Geometry: final body of the model. Coordinates: model frame, mm. A direction names the side the tool comes from. Coordinates: 2 decimals unless noted, no trailing zeros. Order: outer loops, then holes, each group sorted by start corner. A loop starts at its lowest first (then second) coordinate and runs counter-clockwise, first axis right, second up. Notation, with made-up numbers: M -25.75,82 L 4.25,82 A15 ccw 4.25,101 Z; hole C 42.25,-23 d11. An arc over 180 degrees is marked long. Use CSV: the item, a comma, the result in double quotes. Start each with the question number.
1. Section query B-B on z = 33. Return the cut outline in (x, y).
2. Set-up query: faces 4 (the flat face through (27.94, 0, 36)), 5 (the flat face through (-29, 52.07, 34)), 6 (the flat face through (0, -50.8, 18)). Return all of +Z, -Z, +X, -X, +Y, -Y with unobstructed straight access to the full face (end or side cutting, diameter ignored); none if empty.
3. Section query C-C on y = 42. Return the cut outline in (x, z).
4. Pull-direction query (Y, two-part tool) for faces 1 (the flat face through (0, 50.8, 18)), 2 (the cylindrical face through (30.301, 55.622, 16.097)), 3 (the flat face through (0, -57.15, 16)); classes: pulls with the +Y half, pulls with the -Y half, needs draft (parallel to the pull), parting line crosses it, or undercut.
5. Material intervals for line 1 (Y direction, x = 0, z = 24); line 2 (X direction, y = -15, z = 17); line 3 (Y direction, x = 21, z = 28), sorted ascending.
6. Section query D-D on x = -15.5. Return the cut outline in (y, z).
7. First-contact query: P1, Ø2.5, axis at x = 5, y = 54.5, coming from the +Z side; P2, Ø1.9, axis at x = -30, z = 33, coming from the +Y side; P3, Ø4, axis at x = 30, z = 33.5, coming from the +Y side; P4, Ø4, axis at x = -5, y = 26.5, coming from the -Z side. Flat tips, straight axial feed; report the tip coordinate or a pass-through.
8. Section query A-A on z = 25. Return the cut outline in (x, y), and give its area (3 significant figures).
from build123d import *

# Parameters (mm, degrees)
F0_W      = 63.5
F0_H      = 114.3
F1_DEPTH  = 31.75
F2_W      = 50.8
F2_H      = 101.6
F3_DEPTH  = 25.4
F4_W      = 12.7
F4_H      = 76.2
F5_DEPTH  = 25.4
F6_R      = 5.08
F7_SIZE   = 2.54
F8_R      = 5.08
F9_R      = 5.08
F10_W     = 6.35
F10_H     = 105.41
F10_W_2   = 3.81
F11_DEPTH = 8.89
F12_R     = 5.08


with BuildPart() as f1:
    # F0 (on Top) → F1 (new body)
    with BuildSketch(Plane.XY):
        Rectangle(F0_W, F0_H)
    extrude(amount=F1_DEPTH)

    # F2 (on face) → F3 (cut)
    with BuildSketch(Plane.XY.offset(31.75)):
        Rectangle(F2_W, F2_H)
    extrude(amount=-F3_DEPTH, mode=Mode.SUBTRACT)

    # F4 (on face) → F5 (join)
    with BuildSketch(Plane.XY.offset(6.35)):
        Rectangle(F4_W, F4_H)
    extrude(amount=F5_DEPTH)

    # F6
    f6_edges = [f1.edges().sort_by_distance(p)[0] for p in [
        (6.35, -38.1, 19.05),
        (-6.35, -38.1, 19.05),
        (6.35, 38.1, 19.05),
        (-6.35, 38.1, 19.05),
    ]]
    fillet(f6_edges, radius=F6_R)

    # F7
    f7_edges = [f1.edges().sort_by_distance(p)[0] for p in [
        (-25.4, 0, 6.35),
        (0, 50.8, 31.75),
        (25.4, 0, 31.75),
        (0, -50.8, 31.75),
    ]]
    chamfer(f7_edges, length=F7_SIZE)

    # F8
    f8_edges = [f1.edges().sort_by_distance(p)[0] for p in [
        (6.35, 0, 31.75),
        (-6.35, 0, 31.75),
    ]]
    fillet(f8_edges, radius=F8_R)

    # F9
    f9_edges = [f1.edges().sort_by_distance(p)[0] for p in [
        (-31.75, -57.15, 15.875),
        (31.75, -57.15, 15.875),
        (31.75, 57.15, 15.875),
        (-31.75, 57.15, 15.875),
    ]]
    fillet(f9_edges, radius=F9_R)

    # F10 (on face) → F11 (join)
    with BuildSketch(Plane.XY.offset(31.75)):
        with Locations((-28.575, -0.635)):
            Rectangle(F10_W, F10_H)
        with Locations((29.845, 0.635)):
            Rectangle(F10_W_2, F10_H)
    extrude(amount=F11_DEPTH)

    # F12
    f12_edges = [f1.edges().sort_by_distance(p)[0] for p in [
        (-28.575, -53.34, 40.64),
        (29.845, -52.07, 40.64),
        (-28.575, 52.07, 40.64),
        (29.845, 53.34, 40.64),
    ]]
    fillet(f12_edges, radius=F12_R)


solid = f1.part
Results list:
1,outline,"M -31.75,-53.34 L -25.4,-53.34 L -25.4,52.07 L -31.75,52.07 Z; M 27.94,-52.07 L 31.75,-52.07 L 31.75,53.34 L 27.94,53.34 Z"
2,face 4,"+Z, +Y, -Y"
2,face 5,"+Z, -X, +Y"
2,face 6,"+Z"
3,outline,"M -31.75,0 L 31.75,0 L 31.75,40.64 L 27.94,40.64 L 27.94,31.75 L 25.4,29.21 L 25.4,6.35 L -22.86,6.35 L -25.4,8.89 L -25.4,40.64 L -31.75,40.64 Z"
4,face 1,"undercut"
4,face 2,"pulls with the +Y half"
4,face 3,"pulls with the -Y half"
5,line 1,"y = -57.15 to -50.8, -38.1 to 38.1, 50.8 to 57.15"
5,line 2,"x = -31.75 to -25.4, -6.35 to 6.35, 25.4 to 31.75"
5,line 3,"y = -57.15 to -50.8, 50.8 to 57.15"
6,outline,"M -57.15,0 L 57.15,0 L 57.15,31.75 L 53.34,31.75 L 50.8,29.21 L 50.8,6.35 L -50.8,6.35 L -50.8,29.21 L -53.34,31.75 L -57.15,31.75 Z"
7,P1,"stops at z = 31.75"
7,P2,"stops at y = 52.07"
7,P3,"stops at y = 56.57"
7,P4,"stops at z = 0"
8,outline,"M -31.75,-52.07 A5.08 ccw -26.67,-57.15 L 26.67,-57.15 A5.08 ccw 31.75,-52.07 L 31.75,52.07 A5.08 ccw 26.67,57.15 L -26.67,57.15 A5.08 ccw -31.75,52.07 Z; M -6.35,-33.02 A5.08 ccw -1.27,-38.1 L 1.27,-38.1 A5.08 ccw 6.35,-33.02 L 6.35,33.02 A5.08 ccw 1.27,38.1 L -1.27,38.1 A5.08 ccw -6.35,33.02 Z; hole M -25.4,-50.8 L 25.4,-50.8 L 25.4,50.8 L -25.4,50.8 Z"
8,area,"3,020 mm²"
